```python
from build123d import *

# Parameters (mm, degrees)
F1_DEPTH = 36.322
F3_DEPTH = 8.382
F4_R     = 4.21986
F5_DEPTH = 46.736


with BuildPart() as f1:
    # F0 (on Front) → F1 (new body)
    with BuildSketch(Plane.XZ):
        Polygon((-14.847217, 24.653712), (-37.392989, 24.287116), (-37.392989, -14.572268), (9.348247, -14.572268), align=None)
    extrude(amount=F1_DEPTH)

    # F2 (on Front) → F3 (join)
    with BuildSketch(Plane.XZ):
        Polygon((-37.069924, 28.770359), (-37.069924, 24.735801), (-36.900819, -14.487034), (9.12904, -14.487034), (15.986776, -14.487034), (-13.213245, 28.770359), align=None)
    extrude(amount=F3_DEPTH)

    # F4 (on Right) → F5 (cut)
    with BuildSketch(Plane.YZ):
        with Locations((-22.545774, 7.057011)):
            Circle(F4_R)
    extrude(amount=-F5_DEPTH, mode=Mode.SUBTRACT)


solid = f1.part
```
Check sheet for the modelled part. Datum: model origin and axes. Units: mm. A direction names the side the tool comes from. Coordinates: 2 decimals unless noted, no trailing zeros. Order: outer loops, then holes, each group sorted by start corner. A loop starts at its lowest first (then second) coordinate and runs counter-clockwise, first axis right, second up. Notation, with made-up numbers: (56, 33.25) -> (70, 33.25) arc R19 ccw to (70, 50.25) -> close; hole circle Ø6 at (47, -39). An arc over 180 degrees is marked (long way). Write item = value, one per line. Start each with the question number.
1) Cross-section at B-B (x = -12). Enter the section's corners in (y, z).
2) Go/stop test with flat-tipped pins: P1, Ø10, axis at y = -31.5, z = 16, coming from the +X side; P2, Ø1, axis at x = -27.5, y = -25.5, coming from the +Z side; P3, Ø10, axis at x = -5.5, y = -16.5, coming from the +Z side; P4, Ø5, axis at y = -22.55, z = 7.06, coming from the -X side. Record where each tip stops, or that it passes through.
3) Material ranges on L1, parallel to X at y = -9, z = -4; L2, parallel to Y at x = 4, z = -4.5; L3, parallel to X at y = -4.5, z = 2, recorded low to high.
4) Cross-section at A-A (y = -20). Enter the section's corners in (x, z), then the cut area to 3 significant figures.
5) Cross-section at C-C (z = 8.5). Enter the section's corners in (x, y).
6) Access from +Z, -Z, +X, -X, +Y, -Y to the whole of each face (thin tool, end or side, straight path). Record for faces 5 (the flat face through (13, -4, -14.487)), 6 (the flat face through (-37.393, -18, 5)).
7) Mould release check, pull along Y, two halves, no side actions. Record for faces 1 (the flat face through (-6.7, -8.382, 12)), 2 (the flat face through (-37.07, -4, 27)), 3 (the cylindrical face through (-19.14, -23.461, 2.937)), 4 (the flat face through (-17, 0, 3)): +Y half, -Y half, draft (parallel to the pull), parting line (faces both ways), or undercut.
8) Cross-section at D-D (x = -3). Enter the section's corners in (y, z).
Ans:
q1.outline = (-36.32, -14.57) -> (0, -14.57) -> (0, 26.97) -> (-8.38, 26.97) -> (-8.38, 20.04) -> (-36.32, 20.04) -> close; hole circle Ø8.44 at (-22.55, 7.06)
q2.P1 = -6.43
q2.P2 = 24.46
q2.P3 = 17.61
q2.P4 = through
q3.L1 = -37.39 to 2.83
q3.L2 = -8.38 to 0
q3.L3 = -37.39 to 4.86
q4.outline = (-37.39, -14.57) -> (9.35, -14.57) -> (-1.92, 3.69) -> (-37.39, 3.69) -> close; (-37.39, 10.42) -> (-6.07, 10.42) -> (-14.85, 24.65) -> (-37.39, 24.29) -> close
q4.area = 1,130 mm²
q5.outline = (-37.39, -36.32) -> (-4.88, -36.32) -> (-4.88, -26.51) -> (-37.39, -26.51) -> close; (-37.39, -18.58) -> (-4.88, -18.58) -> (-4.88, -8.38) -> (0.47, -8.38) -> (0.47, 0) -> (-37.39, 0) -> close
q6.face_5 = -Z, +X, +Y, -Y
q6.face_6 = +Z, -Z, -X, +Y, -Y
q7.face_1 = -Y half
q7.face_2 = draft
q7.face_3 = undercut
q7.face_4 = +Y half
q8.outline = (-36.32, -14.57) -> (0, -14.57) -> (0, 13.64) -> (-8.38, 13.64) -> (-8.38, 5.45) -> (-18.65, 5.45) arc R4.22 cw to (-26.45, 5.45) -> (-36.32, 5.45) -> close
